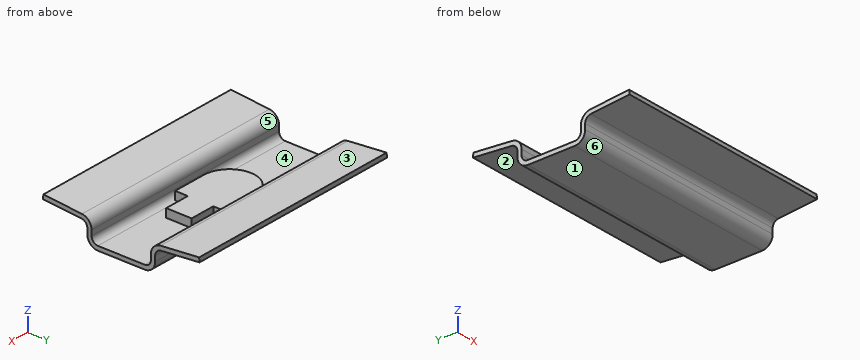
```python
from build123d import *

# Parameters (mm, degrees)
BASE_FLANGE1_DEPTH  = 13
BOSS_EXTRUDE2_DEPTH = 1


# Sheet-metal steps are written as plain solids
with BuildPart() as part:
    # Sketch1 → Base-Flange1 (new, symmetric)
    with BuildSketch(Plane.YZ):
        with BuildLine():
            Line((-9.23, 3), (-4.67240108, 2.601261762))
            ThreePointArc((-4.67240108, 2.601261762), (-4.193521514, 2.365104494), (-4, 1.867464747))
            Line((-4, 1.867464747), (-4, 1.2366))
            ThreePointArc((-4, 1.2366), (-3.637808246, 0.362191754), (-2.7634, 0))
            Line((-2.7634, 0), (2.7634, 0))
            ThreePointArc((2.7634, 0), (3.637808246, 0.362191754), (4, 1.2366))
            Line((4, 1.2366), (4, 1.867464747))
            ThreePointArc((4, 1.867464747), (4.193521514, 2.365104494), (4.67240108, 2.601261762))
            Line((4.67240108, 2.601261762), (9.23, 3))
            Line((9.23, 3), (9.186422129, 3.498097349))
            Line((9.186422129, 3.498097349), (4.628823209, 3.099359111))
            ThreePointArc((4.628823209, 3.099359111), (3.824882845, 2.702899598), (3.5, 1.867464747))
            Line((3.5, 1.867464747), (3.5, 1.2366))
            ThreePointArc((3.5, 1.2366), (3.284254855, 0.715745145), (2.7634, 0.5))
            Line((2.7634, 0.5), (-2.7634, 0.5))
            ThreePointArc((-2.7634, 0.5), (-3.284254855, 0.715745145), (-3.5, 1.2366))
            Line((-3.5, 1.2366), (-3.5, 1.867464747))
            ThreePointArc((-3.5, 1.867464747), (-3.824882845, 2.702899598), (-4.628823209, 3.099359111))
            Line((-4.628823209, 3.099359111), (-9.186422129, 3.498097349))
            Line((-9.186422129, 3.498097349), (-9.23, 3))
        make_face()
    extrude(amount=BASE_FLANGE1_DEPTH, both=True)

    # Sketch6 → Boss-Extrude2 (add)
    with BuildSketch(Plane.XY.offset(0.5)):
        with BuildLine():
            Line((-2, 3), (2, 3))
            Line((2, 3), (2, 1.5))
            Line((2, 1.5), (5, 1.5))
            Line((5, 1.5), (5, -1.5))
            Line((5, -1.5), (2, -1.5))
            Line((2, -1.5), (2, -3))
            Line((2, -3), (-2, -3))
            ThreePointArc((-2, -3), (-5, 0), (-2, 3))
        make_face()
    extrude(amount=BOSS_EXTRUDE2_DEPTH)


solid = part.part
```
Check sheet for the modelled part. Datum: model origin and axes. Units: mm. Face numbers are marked on the shaded views. A direction names the side the tool comes from. Coordinates: 2 decimals unless noted, no trailing zeros. Write each loop counter-clockwise with the first axis right and the second up, starting at its lowest first coordinate (ties: lowest second). Pieces come first, ordered by that corner, then holes. Notation, with made-up numbers: M -23,53 L 31,53 A16 ccw 31,67 Z; hole C 9,-18.5 d1. An arc over 180 degrees is marked long. Use one line per item in the form item = value.
Item 1: Sectioned sample at C-C, the plane x = 10.25. Record the cut outline in (y, z), and give its area (3 significant figures).
Answer below:
outline = M -9.23,3 L -4.67,2.6 A0.74 cw -4,1.87 L -4,1.24 A1.24 ccw -2.76,0 L 2.76,0 A1.24 ccw 4,1.24 L 4,1.87 A0.74 cw 4.67,2.6 L 9.23,3 L 9.19,3.5 L 4.63,3.1 A1.24 ccw 3.5,1.87 L 3.5,1.24 A0.74 cw 2.76,0.5 L -2.76,0.5 A0.74 cw -3.5,1.24 L -3.5,1.87 A1.24 ccw -4.63,3.1 L -9.19,3.5 Z
area = 11.0 mm^2
Item 2: Sectioned sample at A-A, the plane x = 3.75. Record the cut outline in (y, z).
Answer below:
outline = M -9.23,3 L -4.67,2.6 A0.74 cw -4,1.87 L -4,1.24 A1.24 ccw -2.76,0 L 2.76,0 A1.24 ccw 4,1.24 L 4,1.87 A0.74 cw 4.67,2.6 L 9.23,3 L 9.19,3.5 L 4.63,3.1 A1.24 ccw 3.5,1.87 L 3.5,1.24 A0.74 cw 2.76,0.5 L 1.5,0.5 L 1.5,1.5 L -1.5,1.5 L -1.5,0.5 L -2.76,0.5 A0.74 cw -3.5,1.24 L -3.5,1.87 A1.24 ccw -4.63,3.1 L -9.19,3.5 Z
Item 3: Sectioned sample at B-B, the plane y = 0. Record the cut outline in (x, z), and give its area (3 significant figures).
Answer below:
outline = M -13,0 L 13,0 L 13,0.5 L 5,0.5 L 5,1.5 L -5,1.5 L -5,0.5 L -13,0.5 Z
area = 23.0 mm^2
Item 4: Sectioned sample at D-D, the plane y = -5.25. Record the cut outline in (x, z), and give its area (3 significant figures).
Answer below:
outline = M -13,2.65 L 13,2.65 L 13,3.15 L -13,3.15 Z
area = 13.0 mm^2
Item 5: Set-up check for the marked faces 4, 5 and 6: record each of +Z, -Z, +X, -X, +Y, -Y from which the full face is reachable in a straight line by a thin tool's end or side.
Answer below:
face_4 = +Z, -X
face_5 = +Z, +X, -X
face_6 = -Z, +X, -X, -Y
Item 6: Release check for a two-part mould opening along Y. For the marked faces 1, 2 and 3 record: pulls with the +Y half, pulls with the -Y half, needs draft (parallel to the pull), parting line crosses it, or undercut.
Answer below:
face_1 = needs draft
face_2 = pulls with the +Y half
face_3 = undercut
Item 7: Material ranges on L1, parallel to Y at x = -11.5, z = 1.5; L2, parallel to Y at x = -11.25, z = 2.5; L3, parallel to Z at x = -11, y = -0.75, recorded low to high. Write a range as from..to.
Answer below:
L1 = -4..-3.5, 3.5..4
L2 = -4.36..-3.67, 3.67..4.36
L3 = 0..0.5
Item 8: Gauge pin test, flat ends, axial feed: pin 1 Ø0.5 at (x, z) = (4, 1) entering from +Y; pin 2 Ø4.5 at (x, y) = (7.5, -1) entering from +Z; pin 3 Ø1.5 at (x, y) = (9, 7) entering from +Z. Record the tip position at first contact, or that the pin passes through.
Answer below:
pin_1 = 4
pin_2 = 0.68
pin_3 = 3.37
